Can you work these out from the model? Positions are in its coordinate system, mm. Face numbers are marked on the shaded views. A direction names the side the tool comes from. Round coordinates to 2 decimals unless told otherwise and drop trailing zeros. Loops run counter-clockwise (first coordinate to the right, second up) from the corner with the lowest first, then second, coordinate; pieces in that order, holes last.
```python
from build123d import *

# Parameters (mm, degrees)
BOSS_EXTRU_1_DEPTH         = 20
BOSS_EXTRU_2_START         = 10
BOSS_EXTRU_2_DEPTH         = 10
CONG_4_R                   = 10
PER_AGEAVANC_1_START       = 12.70456624
PER_AGEAVANC_1_OUTLINE_R   = 3.5
PER_AGEAVANC_1_DEPTH       = 5.79543376
PER_AGEAVANC_1_START_2     = 18.5
PER_AGEAVANC_1_2_OUTLINE_R = 1.7
PER_AGEAVANC_1_2_DEPTH     = 2
CONG_6_R                   = 1


# Read off the part's stored shape, not the designer's step: PerçageAvancé1
with BuildPart() as part:
    # Esquisse4 → Boss.-Extru.1 (new body)
    with BuildSketch(Plane(origin=(0, 0, 0), x_dir=(1, 0, 0), z_dir=(0, 1, 0))):
        with BuildLine():
            Line((-25.402205763, -20.5), (-25.402205763, -18.5))
            Line((-25.402205763, -18.5), (-20.402205763, -18.5))
            ThreePointArc((-20.402205763, -18.5), (0, 0), (20.402205763, -18.5))
            Line((20.402205763, -18.5), (25.402205763, -18.5))
            Line((25.402205763, -18.5), (25.402205763, -20.5))
            Line((25.402205763, -20.5), (18.5, -20.5))
            ThreePointArc((18.5, -20.5), (0, -2), (-18.5, -20.5))
            Line((-18.5, -20.5), (-25.402205763, -20.5))
        make_face()
    extrude(amount=BOSS_EXTRU_1_DEPTH)

    # Esquisse8 → Boss.-Extru.2 (add)
    with BuildSketch(Plane.XZ.offset(BOSS_EXTRU_2_START)):
        with BuildLine():
            Line((-25.402205763, 20.5), (-15, 20.5))
            ThreePointArc((-15, 20.5), (0, 5.5), (15, 20.5))
            Line((15, 20.5), (25.402205763, 20.5))
            Line((25.402205763, 20.5), (25.402205763, 18.5))
            Line((25.402205763, 18.5), (20.402205763, 18.5))
            ThreePointArc((20.402205763, 18.5), (0, 0), (-20.402205763, 18.5))
            Line((-20.402205763, 18.5), (-25.402205763, 18.5))
            Line((-25.402205763, 18.5), (-25.402205763, 20.5))
        make_face()
    extrude(amount=-BOSS_EXTRU_2_DEPTH)

    # Congé4
    # the kernel refuses this fillet: 10 mm, written as the material it adds along each edge
    with BuildSketch(Plane(origin=(20.402205763, 20, 18.5), x_dir=(1, 0, 0), z_dir=(0, -1, 0))) as cong_4_piece_1:
        with BuildLine():
            CenterArc((7.806559521, -9.598084374), CONG_4_R, 106.29935787, 51.350539993)
            Line((-1.442215982, -5.79543376), (-1.627191492, -5.719380747))
            ThreePointArc((-1.627191492, -5.719380747), (-0.703011933, -2.902220154), (-0.19904591, 0.019512195))
            Line((-0.19904591, 0.019512195), (0, 0.2))
            ThreePointArc((0, 0.2), (2.5, 0.2), (4.94386881, 0.191961687))
            Line((4.94386881, 0.191961687), (5, 0))
        make_face()
    extrude(amount=30)
    with BuildSketch(Plane(origin=(-20.402205763, 20, 18.5), x_dir=(0.241488677516522, 0, -0.9704036369631562), z_dir=(0, -1, 0))) as cong_4_piece_2:
        with BuildLine():
            CenterArc((7.42882025, -9.893342453), CONG_4_R, 98.375682161, 51.350539993)
            Line((-1.207443388, -4.852018185), (-1.38016866, -4.751191699))
            ThreePointArc((-1.38016866, -4.751191699), (-0.797802421, -2.377711357), (-0.194080727, 0.048297736))
            Line((-0.194080727, 0.048297736), (0.029132628, 0.197866849))
            ThreePointArc((0.029132628, 0.197866849), (2.986094414, -0.01864797), (5.9430562, 0.197866849))
            Line((5.9430562, 0.197866849), (5.972188828, 0))
        make_face()
    extrude(amount=30)

    # PerçageAvancé1 outline → PerçageAvancé1 (cut)
    with BuildSketch(Plane.XY.offset(PER_AGEAVANC_1_START)):
        with BuildLine():
            Line((27, 15.818747829), (25.402205763, 17.449489743))
            ThreePointArc((25.402205763, 17.449489743), (19.402205763, 15), (25.402205763, 12.550510257))
            Line((25.402205763, 12.550510257), (27, 14.181252171))
            Line((27, 14.181252171), (27, 15.818747829))
        make_face()
        with BuildLine():
            Line((-25.402205763, 17.449489743), (-27, 15.818747829))
            Line((-27, 15.818747829), (-27, 14.181252171))
            Line((-27, 14.181252171), (-25.402205763, 12.550510257))
            ThreePointArc((-25.402205763, 12.550510257), (-19.402205763, 15), (-25.402205763, 17.449489743))
        make_face()
        with Locations((21.460868066, -5)):
            Circle(PER_AGEAVANC_1_OUTLINE_R)
        with Locations((-21.460868066, -5)):
            Circle(PER_AGEAVANC_1_OUTLINE_R)
    extrude(amount=PER_AGEAVANC_1_DEPTH, mode=Mode.SUBTRACT)

    # Per_ageAvanc_1 2 outline → Per_ageAvanc_1 2 (cut)
    with BuildSketch(Plane.XY.offset(PER_AGEAVANC_1_START_2)):
        with Locations((22.902205763, 15)):
            Circle(PER_AGEAVANC_1_2_OUTLINE_R)
        with Locations((21.460868066, -5)):
            Circle(PER_AGEAVANC_1_2_OUTLINE_R)
        with Locations((-21.460868066, -5)):
            Circle(PER_AGEAVANC_1_2_OUTLINE_R)
        with Locations((-22.902205763, 15)):
            Circle(PER_AGEAVANC_1_2_OUTLINE_R)
    extrude(amount=PER_AGEAVANC_1_2_DEPTH, mode=Mode.SUBTRACT)

    # Congé6
    # the kernel refuses this fillet: 1 mm, written as the material it takes off along each edge
    with BuildSketch(Plane(origin=(25.402205763, -12.5, 20.5), x_dir=(-1, 0, 0), z_dir=(0, 1, 0))) as cong_6_piece_1:
        with BuildLine():
            CenterArc((CONG_6_R, -CONG_6_R), CONG_6_R, 90, 90)
            Line((0, -CONG_6_R), (0, 0))
            Line((0, 0), (CONG_6_R, 0))
        make_face()
    extrude(amount=35, mode=Mode.SUBTRACT)
    with BuildSketch(Plane(origin=(18.5, 0, 20.5), x_dir=(-0.02564946435665691, 0, -0.9996709983680714), z_dir=(0, 1, 0))) as cong_6_piece_2:
        with BuildLine():
            CenterArc((0.974679646, -0.999670998), CONG_6_R, 91.469767243, 87.060465514)
            Line((-0.024991353, -0.974021534), (0, 0))
            ThreePointArc((0, 0), (0.474515091, -0.00608653), (0.949030181, 0))
        make_face()
    extrude(amount=22.435855235, mode=Mode.SUBTRACT)
    with BuildSketch(Plane(origin=(-18.5, 0, 20.5), x_dir=(-1, 0, 0), z_dir=(0, 1, 0))) as cong_6_piece_3:
        with BuildLine():
            CenterArc((0.974342094, -1), CONG_6_R, 90, 87.060465514)
            ThreePointArc((-0.024342116, -0.948717949), (-0.00608653, -0.474515091), (0, 0))
            Line((0, 0), (0.974342094, 0))
        make_face()
    extrude(amount=22.435855235, mode=Mode.SUBTRACT)
    with BuildSketch(Plane(origin=(-25.402205763, 22.5, 20.5), x_dir=(0, 0, -1), z_dir=(0, -1, 0))) as cong_6_piece_4:
        with BuildLine():
            CenterArc((CONG_6_R, CONG_6_R), CONG_6_R, 180, 90)
            Line((0, CONG_6_R), (0, 0))
            Line((0, 0), (CONG_6_R, 0))
        make_face()
    extrude(amount=35, mode=Mode.SUBTRACT)
    with BuildSketch(Plane(origin=(15, -12.421798557, 20.5), x_dir=(1, 0, 0), z_dir=(0, 1, 0))) as cong_6_piece_5:
        with BuildLine():
            CenterArc((0.968719423, 1), CONG_6_R, 183.583321698, 86.416678302)
            ThreePointArc((-0.029325541, 0.9375), (-0.007333178, 0.468979274), (0, 0))
            Line((0, 0), (0.968719423, 0))
        make_face()
    extrude(amount=14.843597113, mode=Mode.SUBTRACT)
    with BuildSketch(Plane(origin=(-15, -12.421798557, 20.5), x_dir=(-1, 0, 0), z_dir=(0, 1, 0))) as cong_6_piece_6:
        with BuildLine():
            CenterArc((0.968719423, -1), CONG_6_R, 90, 86.416678302)
            ThreePointArc((-0.029325541, -0.9375), (-0.007333178, -0.468979274), (0, 0))
            Line((0, 0), (0.968719423, 0))
        make_face()
    extrude(amount=14.843597113, mode=Mode.SUBTRACT)


solid = part.part
```
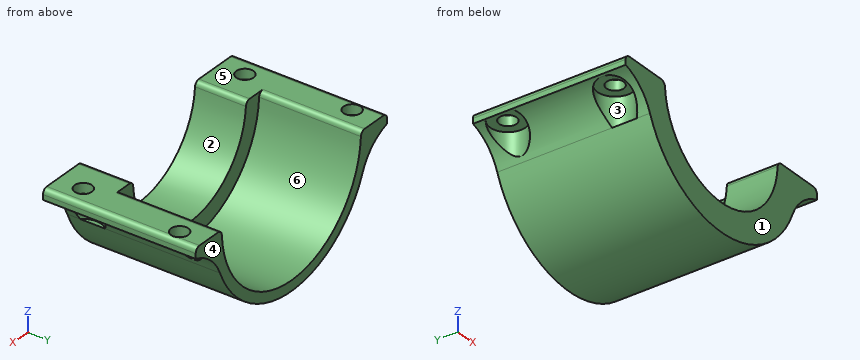
(1) Suppose I cut it at A-A (z = 19). Write out the boundary of the cut face in (x, y), then the cut area to 3 significant figures.
(2) For pin 1 (5 mm diameter, centred on x = 23, y = 16.5, fed in from -Z); pin 2 (2 mm diameter, centred on x = -21.46, y = -5, fed in from -Z); pin 3 (1.5 mm diameter, centred on x = 8.5, y = 11, fed in from +Z); pin 4 (4 mm diameter, centred on x = 5, y = 9.5, fed in from +Z), each with a flat end and sliding along its axis, tell me the tip position at first contact or that it passes through.
(3) Suppose I cut it at D-D (x = 0). Write out the boundary of the cut face in (y, z), then the cut area to 3 significant figures.
(4) Which directions (+Z, -Z, +X, -X, +Y, -Y) give clear straight access to the entire face, cutting with the end or side of a thin tool? Please do the marked faces 5 and 6.
(5) If I drill on line 1 (X direction, y = 4, z = 16); line 2 (Y direction, x = 3, z = 4); line 3 (X direction, y = 12.5, z = 3.5), over which ranges is the centre line in solid material (lowest first)?
(6) We'd pull the mould along Y, two halves only. Please class the marked faces 1, 2, 3 and 4: released by +Y, released by -Y, zero draft, split by the parting line, or undercut.
(7) Suppose I cut it at B-B (x = -20.5). Write out the boundary of the cut face in (y, z), then the cut area to 3 significant figures.
Check result:
1. outline: (-25.4, -10) - (-14.92, -10) - (-14.92, 0) - (-18.44, 0) - (-18.44, 20) - (-25.4, 20) - close; (14.92, -10) - (25.4, -10) - (25.4, 20) - (18.44, 20) - (18.44, 0) - (14.92, 0) - close; hole circle Ø3.4 at (-22.9, 15); hole circle Ø3.4 at (-21.46, -5); hole circle Ø3.4 at (21.46, -5); hole circle Ø3.4 at (22.9, 15)
1. area: 452 mm2
2. pin 1: stops at z = 15.75
2. pin 2: passes through
2. pin 3: stops at z = 4.48
2. pin 4: stops at z = 3.38
3. outline: (-10, 0) - (20, 0) - (20, 2) - (0, 2) - (0, 5.5) - (-10, 5.5) - close
3. area: 95.0 mm2
4. face 5: +Z, +X, -X, +Y, -Y
4. face 6: +Z, +Y
5. line 1: x = -21.16 to -17.94, 17.94 to 21.16
5. line 2: y = -10 to 0
5. line 3: x = -11.46 to -7.3, 7.3 to 11.46
6. face 1: released by -Y
6. face 2: zero draft
6. face 3: undercut
6. face 4: released by +Y
7. outline: (-10, 15.27) - (-8.37, 15.27) - (-8.37, 18.5) - (-6.4, 18.5) - (-6.4, 20.5) - (-10, 20.5) - close; (-3.6, 18.5) - (-1.63, 18.5) - (-1.63, 15.27) - (12.45, 15.27) - (12.45, 18.5) - (17.55, 18.5) - (17.55, 15.27) - (20, 15.27) - (20, 20.5) - (-3.6, 20.5) - close
7. area: 113 mm2
